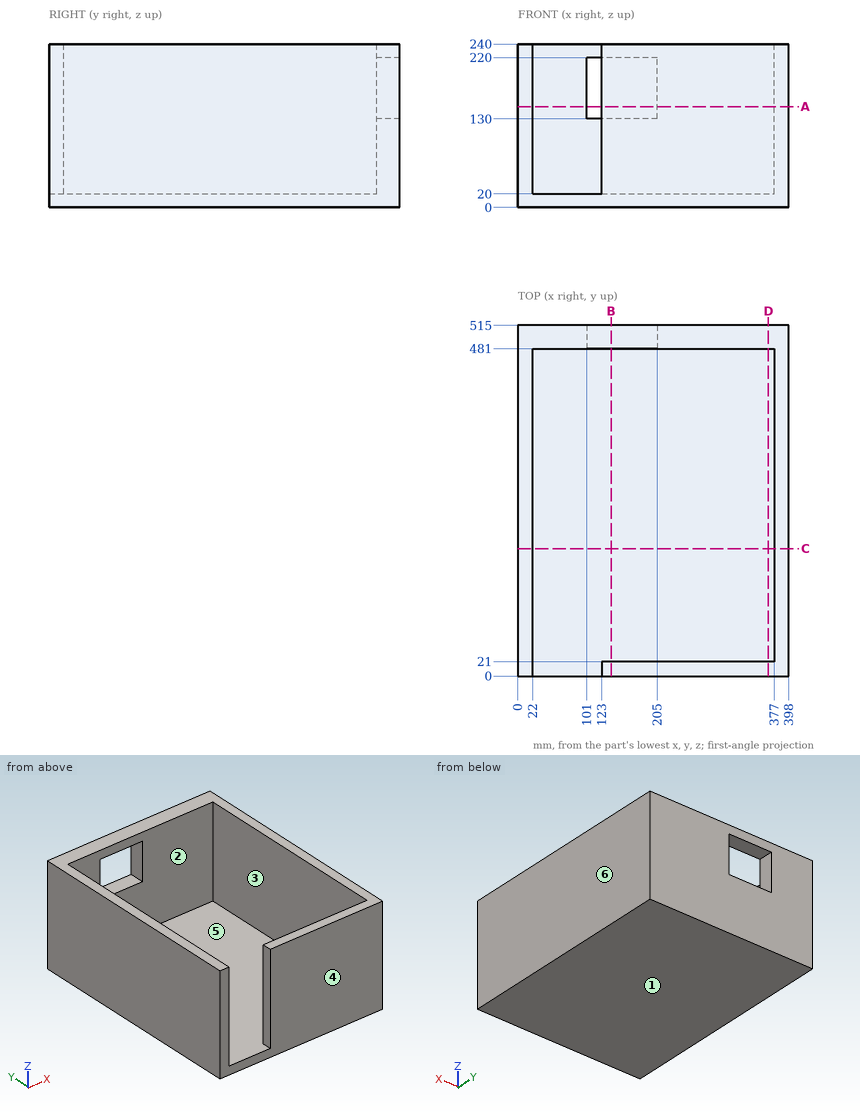
Verification items for this drawing (mm, ordinates from the low corner). A direction names the side the tool comes from. Coordinates: 2 decimals unless noted, no trailing zeros. Write each loop counter-clockwise with the first axis right and the second up, starting at its lowest first coordinate (ties: lowest second). Pieces come first, ordered by that corner, then holes. Notation, with made-up numbers: (46.5, -20) -> (104.5, -20) arc R21 cw to (104.5, 10) -> close; hole circle Ø11 at (-1, 17.5). An arc over 180 degrees is marked (long way). Use CSV: the item, a comma, the result in double quotes. Start each with the question number.
Item 1: Cross-section at A-A, the plane z = 148. Record the cut outline in (x, y), plus the area to 3 significant figures.
Item 2: Depth check by flat-ended pin: pin 1 Ø6 at (x, y) = (343.5, 91) entering from +Z. Enter the tip coordinate at first touch or a pass-through.
Item 3: Mould release check, pull along X, two halves, no side actions. Record for the marked faces 3, 4, 5 and 6: released by +X, released by -X, zero draft, split by the parting line, or undercut.
Item 4: Set-up check for the marked faces 1 and 2: record each of +Z, -Z, +X, -X, +Y, -Y from which the full face is reachable in a straight line by a thin tool's end or side.
Item 5: Cross-section at C-C, the plane y = 187. Record the cut outline in (x, z), plus the area to 3 significant figures.
Item 6: Thickness scan on line 1 (X direction, y = 147.5, z = 102); line 2 (Y direction, x = 148, z = 20.5); line 3 (Z direction, x = 309, y = 78.5). Record the ranges inside material, lowest first.
Item 7: Cross-section at D-D, the plane x = 368. Record the cut outline in (y, z), plus the area to 3 significant figures.
Item 8: Cross-section at B-B, the plane x = 137. Record the cut outline in (y, z), plus the area to 3 significant figures.
Answers:
1,outline,"(0, 0) -> (22, 0) -> (22, 481) -> (101, 481) -> (101, 515) -> (0, 515) -> close; (123, 0) -> (398, 0) -> (398, 515) -> (205, 515) -> (205, 481) -> (377, 481) -> (377, 21) -> (123, 21) -> close"
1,area,"36,000 mm^2"
2,pin 1,"z = 20"
3,face 3,"undercut"
3,face 4,"zero draft"
3,face 5,"undercut"
3,face 6,"released by +X"
4,face 1,"-Z, +X, -X, +Y, -Y"
4,face 2,"+Z"
5,outline,"(0, 0) -> (398, 0) -> (398, 240) -> (377, 240) -> (377, 20) -> (22, 20) -> (22, 240) -> (0, 240) -> close"
5,area,"17,400 mm^2"
6,line 1,"0 to 22, 377 to 398"
6,line 2,"0 to 21, 481 to 515"
6,line 3,"0 to 20"
7,outline,"(0, 0) -> (515, 0) -> (515, 240) -> (481, 240) -> (481, 20) -> (21, 20) -> (21, 240) -> (0, 240) -> close"
7,area,"22,400 mm^2"
8,outline,"(0, 0) -> (515, 0) -> (515, 130) -> (481, 130) -> (481, 20) -> (21, 20) -> (21, 240) -> (0, 240) -> close; (481, 220) -> (515, 220) -> (515, 240) -> (481, 240) -> close"
8,area,"19,300 mm^2"
